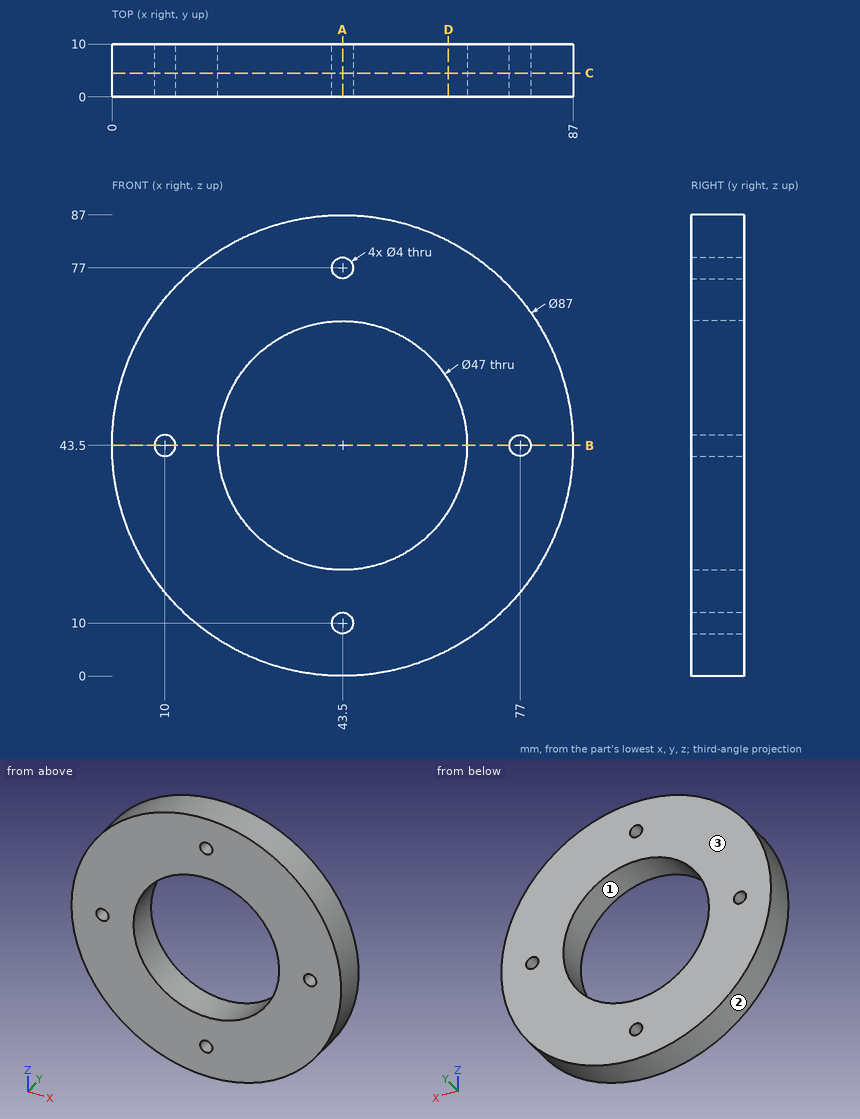
Can you work these out from the drawing? Everything is in mm from the part's minimum corner. Coordinates: 2 decimals unless noted, no trailing zeros. Loops run counter-clockwise (first coordinate to the right, second up) from the corner with the lowest first, then second, coordinate; pieces in that order, holes last. Notation, with made-up numbers: M -32,33.5 L -6,33.5 A20 ccw -6,68.5 Z; hole C 89.25,45 d3. An arc over 180 degrees is marked long. One line per item, written item: value.
1. Please list where these lines run through material, in increasing order: probe 1 along Z at (x, y) = (43.5, 6.5); probe 2 along Z at (x, y) = (54, 0.5); probe 3 along Z at (x, y) = (77, 7.25).
Geometry says:
probe 1: z = 0 to 8, 12 to 20, 67 to 75, 79 to 87
probe 2: z = 1.29 to 22.48, 64.52 to 85.71
probe 3: z = 15.75 to 41.5, 45.5 to 71.25
2. Imagine slicing it at D-D (x = 63.5). List the corners of the cut face in (y, z) for me, and give its area (3 significant figures).
Geometry says:
outline: M 0,4.87 L 10,4.87 L 10,31.16 L 0,31.16 Z; M 0,55.84 L 10,55.84 L 10,82.13 L 0,82.13 Z
area: 526 mm2
3. Imagine slicing it at A-A (x = 43.5). List the corners of the cut face in (y, z) for me, and give its area (3 significant figures).
Geometry says:
outline: M 0,0 L 10,0 L 10,8 L 0,8 Z; M 0,12 L 10,12 L 10,20 L 0,20 Z; M 0,67 L 10,67 L 10,75 L 0,75 Z; M 0,79 L 10,79 L 10,87 L 0,87 Z
area: 320 mm2
4. Imagine slicing it at B-B (z = 43.5). List the corners of the cut face in (x, y) for me, and give its area (3 significant figures).
Geometry says:
outline: M 0,0 L 8,0 L 8,10 L 0,10 Z; M 12,0 L 20,0 L 20,10 L 12,10 Z; M 67,0 L 75,0 L 75,10 L 67,10 Z; M 79,0 L 87,0 L 87,10 L 79,10 Z
area: 320 mm2
5. Will these pins go through, and if not, where does the flat tip stop? pin 1 Ø1 at (x, y) = (19, 6) entering from -Z; pin 2 Ø3.5 at (x, z) = (43.5, 10) entering from -Y; pin 3 Ø3 at (y, z) = (4, 73) entering from +X; pin 4 Ø6 at (y, z) = (8.5, 66.5) entering from -X.
Geometry says:
pin 1: stops at z = 7.22
pin 2: passes through
pin 3: stops at x = 76.79
pin 4: stops at x = 4.87
6. Imagine slicing it at C-C (y = 4.5). List the corners of the cut face in (x, z) for me, and give its area (3 significant figures).
Geometry says:
outline: C 43.5,43.5 d87; hole C 10,43.5 d4; hole C 43.5,43.5 d47; hole C 43.5,10 d4; hole C 43.5,77 d4; hole C 77,43.5 d4
area: 4,160 mm2
7. Thinking about a two-plate mould opening in Z: for the marked faces 1, 2 and 3, which applies, +Z half, -Z half, draft (parallel to the pull), parting line (faces both ways), or undercut?
Geometry says:
face 1: undercut
face 2: parting line
face 3: draft
